Autodesk Inventor part; units mm, degrees
ref_plane "YZ Plane" through (0, 0, 0) normal (1, 0, 0) x (0, 1, 0)
ref_plane "XY Plane" through (0, 0, 0) normal (0, 0, 1) x (1, 0, 0)
sketch "Sketch1" plane through (0, 0, 0) normal (0, 1, 0) x (-1, 0, 0)
  circle A0 centre (0, 0) radius 4
  circle A1 centre (0, 0) radius 2.25
  dimension "d0" = 8
  dimension "d3" = 4.5
extrude "Extrusion1" add sketch "Sketch1" along normal blind 80 contours A0 | A1
extrude "Extrusion2" cut sketch "Sketch1" along normal blind 7
sketch "Sketch2" plane through (0, 0, 0) normal (1, 0, 0) x (0, 1, 0)
  line L0 (80, -4) -> (80, 4)
  circle A0 centre (76, 0) radius 2
  point P0 (0, 0)
  dimension "d6" = 4
  dimension "d7" = 4
extrude "Extrusion3" cut sketch "Sketch2" along normal through all both and the other way through all
thread "Thread1"
fillet "Fillet1" radius 1 2 edges at (4, 80, 0) (2.25, 0, 0)
ref_plane "Work Plane1" through (0, 73, 0) normal (0, 1, 0) x (-1, 0, 0)
ref_plane "Work Plane2" through (0, 7, 0) normal (0, 1, 0) x (-1, 0, 0)
extrude "Extrusion4" cut sketch "Sketch1" along normal blind 4 contours A1
sketch "Sketch3" plane through (0, 4, 0) normal (0, -1, 0) x (1, 0, 0)
  circle A0 centre (0, -0.1147) radius 3.4149
  point P0 (0, 0)
extrude "Extrusion5" add sketch "Sketch3" against normal blind 0.35
fillet "Fillet3" radius 0.2 1 edges at (-3.4149, 4, -0.1147)
properties part number "clampScrew"
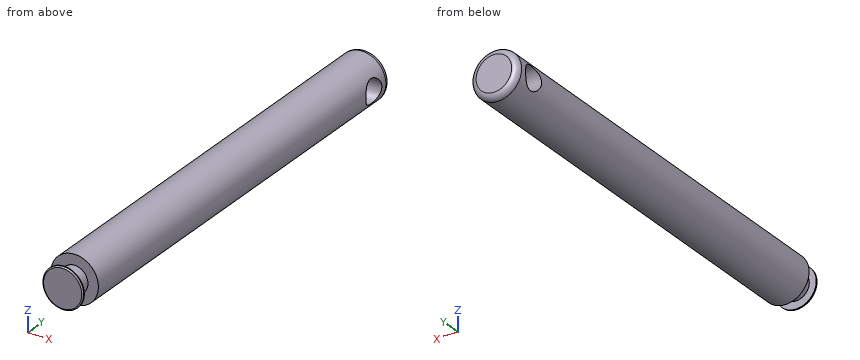
Model file for the job. Use its own axes, mm. Give positions to 0.01 mm unless a question says otherwise; leave off trailing zeros. Order: outer loops, then holes, each group sorted by start corner. A loop starts at its lowest first (then second) coordinate and runs counter-clockwise, first axis right, second up. Notation, with made-up numbers: (69, -32.75) -> (85, -32.75) arc R7 cw to (85, -23.75) -> close; hole circle Ø3 at (55.25, 29). An arc over 180 degrees is marked (long way). Use CSV: the item, a comma, the result in double quotes.
1. Band-saw the part on C-C, the plane y = 64.5. Give the cut face in (x, z).
Outcome:
outline,"circle Ø8 at (0, 0)"
2. Band-saw the part on B-B, the plane y = 76. Give the cut face in (x, z), then the cut area to 3 significant figures.
Outcome:
outline,"(-3.46, -2) arc R4 ccw to (3.46, -2) -> close; (-3.46, 2) -> (3.46, 2) arc R4 ccw to start"
area,"19.7 mm²"
3. Drop flat-ended pins along their axis: pin 1 (1 mm diameter, centred on x = -2, y = 45, fed in from +Z); pin 2 (1.5 mm diameter, centred on y = 52.5, z = -2.5, fed in from +X). Give the stop position or say it passes through.
Outcome:
pin 1,"z = 3.71"
pin 2,"x = 3.6"
4. Band-saw the part on A-A, the plane x = 0. Give the cut face in (y, z).
Outcome:
outline,"(4, -3.33) arc R0.2 ccw to (4.2, -3.53) -> (4.35, -3.53) -> (4.35, -2.25) -> (7, -2.25) -> (7, -4) -> (79, -4) arc R1 ccw to (80, -3) -> (80, 3) arc R1 ccw to (79, 4) -> (7, 4) -> (7, 2.25) -> (4.35, 2.25) -> (4.35, 3.3) -> (4.2, 3.3) arc R0.2 ccw to (4, 3.1) -> close; hole circle Ø4 at (76, 0)"
5. Drill centre lines: line 1 along Y through (x, z) = (-0.5, 2.5); line 2 along Y through (x, z) = (-2.5, -1); line 3 along Y through (x, z) = (0.75, 0). Where is each one in solid material? Low to high. Write a range as from..to.
Outcome:
line 1,"4..4.35, 7..80"
line 2,"4..4.35, 7..74.27, 77.73..80"
line 3,"4..74, 78..80"
